from build123d import *

# Parameters (mm, degrees)
F3_SIZE = 5.08


with BuildPart() as f2:
    # F2: sweep along a path in F1
    with BuildLine(Plane.YZ) as f2_path:
        Line((0, 0), (609.6, 0))
        Line((609.6, 0), (609.6, 228.6))
        Line((609.6, 228.6), (152.4, 228.6))
    # F0 (on Front) → F2 (sweep)
    with BuildSketch(Plane.XZ):
        with BuildLine():
            ThreePointArc((50.8, 44.45), (48.9401280605, 48.9401280605), (44.45, 50.8))
            Line((44.45, 50.8), (-44.45, 50.8))
            ThreePointArc((-44.45, 50.8), (-48.9401280605, 48.9401280605), (-50.8, 44.45))
            Line((-50.8, 44.45), (-50.8, -44.45))
            ThreePointArc((-50.8, -44.45), (-48.9401280605, -48.9401280605), (-44.45, -50.8))
            Line((-44.45, -50.8), (44.45, -50.8))
            ThreePointArc((44.45, -50.8), (48.9401280605, -48.9401280605), (50.8, -44.45))
            Line((50.8, -44.45), (50.8, 44.45))
        make_face()
        with BuildLine():
            Line((-38.1, 44.45), (38.1, 44.45))
            ThreePointArc((38.1, 44.45), (42.5901280605, 42.5901280605), (44.45, 38.1))
            Line((44.45, 38.1), (44.45, -38.1))
            ThreePointArc((44.45, -38.1), (42.5901280605, -42.5901280605), (38.1, -44.45))
            Line((38.1, -44.45), (-38.1, -44.45))
            ThreePointArc((-38.1, -44.45), (-42.5901280605, -42.5901280605), (-44.45, -38.1))
            Line((-44.45, -38.1), (-44.45, 38.1))
            ThreePointArc((-44.45, 38.1), (-42.5901280605, 42.5901280605), (-38.1, 44.45))
        make_face(mode=Mode.SUBTRACT)
    sweep(path=f2_path.line, transition=Transition.RIGHT)

    # F3
    f3_edges = [f2.edges().sort_by_distance(p)[0] for p in [
        (0, 152.4, 279.4),
    ]]
    chamfer(f3_edges, length=F3_SIZE)


solid = f2.part
Could you check a few things on this model? Use its own coordinates, in mm. A direction names the side the tool comes from. Give positions to 0.01 mm unless a question says otherwise; leave off trailing zeros. Order: outer loops, then holes, each group sorted by start corner. A loop starts at its lowest first (then second) coordinate and runs counter-clockwise, first axis right, second up. Notation, with made-up numbers: (-3, 2.5) - (9, 2.5) arc R21 cw to (9, 33.5) - close; hole circle Ø10 at (-0.5, 9.25). An arc over 180 degrees is marked (long way). Return JSON: item names as keys, results as strings. Group by question number.
Q1. Thinking about a two-plate mould opening in Z: for faces 1 (the face through (-1, 335, -50.8)), 2 (the face through (-1, 660.4, 117)), 3 (the face through (1, 400, 273.05)), which applies, pulls with the +Z half, pulls with the -Z half, needs draft (parallel to the pull), parting line crosses it, or undercut?
Q2. Which directions (+Z, -Z, +X, -X, +Y, -Y) give clear straight access to the entire face, cutting with the end or side of a thin tool? Please do faces 4 (the face through (-1, 287, 44.45)), 5 (the face through (-44.45, 400, 11)), 6 (the face through (50.8, 404, 42)), 7 (the face through (1, 355, 177.8)), 8 (the face through (-1, 405, 279.4)).
Q3. Suppose I cut it at C-C, the plane y = 257.5. State how many separate pieces and enclosed holes the cut face has, and give its area (3 significant figures).
Q4. Suppose I cut it at B-B, the plane z = 137.5. Please give me the cut outline in (x, y).
Q5. Will this pin go through, and if not, where does the flat tip stop? pin 1 Ø1 at (x, z) = (19, 69) entering from -Y.
Q6. Please list where these lines run through material, in increasing order: line 1 along Z through (x, y) = (3.5, 176); line 2 along Y through (x, z) = (-16.5, 146). Write a range as [from, to].
Q7. Suppose I cut it at D-D, the plane y = 112. Please give me the cut outline in (x, z), and give its area (3 significant figures).
Q8. Suppose I cut it at A-A, the plane x = -3. Please give me the cut outline in (y, z).
Resolved:
{
 "1": {"face 1": "pulls with the -Z half", "face 2": "needs draft", "face 3": "undercut"},
 "2": {"face 4": "-Y", "face 5": "none", "face 6": "+Z, -Z, +X, +Y, -Y", "face 7": "+X, -X, -Y", "face 8": "+Z, +X, -X, +Y, -Y"},
 "3": {"separate pieces": "2", "enclosed holes": "2", "area": "4,840 mm2"},
 "4": {"outline": "(-50.8, 565.15) arc R6.35 ccw to (-44.45, 558.8) - (44.45, 558.8) arc R6.35 ccw to (50.8, 565.15) - (50.8, 654.05) arc R6.35 ccw to (44.45, 660.4) - (-44.45, 660.4) arc R6.35 ccw to (-50.8, 654.05) - close; hole (-44.45, 571.5) arc R6.35 ccw to (-38.1, 565.15) - (38.1, 565.15) arc R6.35 ccw to (44.45, 571.5) - (44.45, 647.7) arc R6.35 ccw to (38.1, 654.05) - (-38.1, 654.05) arc R6.35 ccw to (-44.45, 647.7) - close"},
 "5": {"pin 1": "stops at y = 558.8"},
 "6": {"line 1": "z = [-50.8, -44.45], [44.45, 50.8], [177.8, 184.15], [273.05, 279.4]", "line 2": "y = [558.8, 565.15], [654.05, 660.4]"},
 "7": {"outline": "(-50.8, -44.45) arc R6.35 ccw to (-44.45, -50.8) - (44.45, -50.8) arc R6.35 ccw to (50.8, -44.45) - (50.8, 44.45) arc R6.35 ccw to (44.45, 50.8) - (-44.45, 50.8) arc R6.35 ccw to (-50.8, 44.45) - close; hole (-44.45, -38.1) arc R6.35 ccw to (-38.1, -44.45) - (38.1, -44.45) arc R6.35 ccw to (44.45, -38.1) - (44.45, 38.1) arc R6.35 ccw to (38.1, 44.45) - (-38.1, 44.45) arc R6.35 ccw to (-44.45, 38.1) - close", "area": "2,420 mm2"},
 "8": {"outline": "(0, -50.8) - (660.4, -50.8) - (660.4, 279.4) - (157.48, 279.4) - (152.4, 274.32) - (152.4, 273.05) - (654.05, 273.05) - (654.05, -44.45) - (0, -44.45) - close; (0, 44.45) - (565.15, 44.45) - (565.15, 184.15) - (152.4, 184.15) - (152.4, 182.88) - (157.48, 177.8) - (558.8, 177.8) - (558.8, 50.8) - (0, 50.8) - close"}
}
